Could you check a few things on this model? Use its own coordinates, in mm. Face numbers are marked on the shaded views. A direction names the side the tool comes from. Round coordinates to 2 decimals unless told otherwise and drop trailing zeros. Loops run counter-clockwise (first coordinate to the right, second up) from the corner with the lowest first, then second, coordinate; pieces in that order, holes last. Notation, with made-up numbers: (39.5, 45.5) -> (66.5, 45.5) arc R20 ccw to (66.5, 72.5) -> close; hole circle Ø10 at (1.25, 38.5). An arc over 180 degrees is marked (long way). Put each result on its own line as item: value. Start each with the question number.
1. I'm going to push flat-ended pins straight in: P1, Ø2, axis at x = 17, z = -3.5, coming from the +Y side; P2, Ø4, axis at y = -1, z = 2, coming from the +X side; P3, Ø8, axis at x = 14.5, y = -13.5, coming from the +Z side; P4, Ø4, axis at x = -0.5, y = 9, coming from the +Z side. Where does each tip first touch, or does it pass through?
2. Imagine slicing it at A-A, the plane x = 0. Please give me the cut outline in (y, z).
3. Imagine slicing it at C-C, the plane z = 3. Please give me the cut outline in (x, y), and give its area (3 significant figures).
4. Imagine slicing it at D-D, the plane x = -6. Please give me the cut outline in (y, z).
5. Which directions (+Z, -Z, +X, -X, +Y, -Y) give clear straight access to the entire face, cutting with the end or side of a thin tool? Please do the marked faces 1, 2 and 3.
6. If we mould it in two halves opening along X, with no side actions, what happens to the marked faces 4, 5 and 6? For each: pulls with the +X half, pulls with the -X half, needs draft (parallel to the pull), parting line crosses it, or undercut.
7. I need wall thicknesses on line 1 (X direction, y = -9, z = -1.5); line 2 (Y direction, x = 0, z = -3.25); line 3 (X direction, y = 7.5, z = -0.75). Which ranges of each line are inside material? Lowest first, please. Write a range as [from, to].
8. Imagine slicing it at B-B, the plane y = 0. Please give me the cut outline in (x, z).
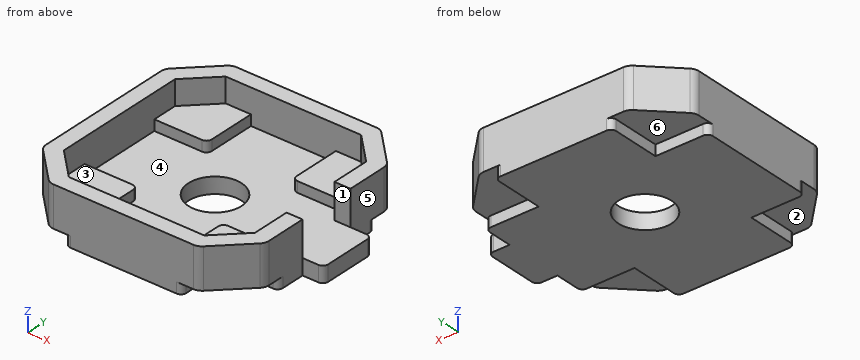
```python
from build123d import *

# Parameters (mm, degrees)
SKETCH1_W           = 42
SKETCH1_H           = 42
BOSS_EXTRUDE1_DEPTH = 4.8
CUT_EXTRUDE1_REACH  = 33.212
CUT_EXTRUDE2_DEPTH  = 2
SKETCH4_W           = 3
SKETCH4_H           = 11
BOSS_EXTRUDE2_DEPTH = 4
SHELL1_T            = -3
CUT_EXTRUDE3_REACH  = 49.202
SKETCH5_W           = 6.6
SKETCH5_H           = 11
CUT_EXTRUDE4_REACH  = 36.032
SKETCH6_R           = 5
FILLET1_R           = 2
FILLET2_R           = 1


with BuildPart() as part:
    # Sketch1 → Boss-Extrude1 (new, symmetric)
    with BuildSketch(Plane.XY):
        Rectangle(SKETCH1_W, SKETCH1_H)
    extrude(amount=BOSS_EXTRUDE1_DEPTH, both=True)

    # Sketch2 → Cut-Extrude1 (cut, up to next)
    with BuildSketch(Plane.XY.offset(4.8), mode=Mode.PRIVATE) as cut_extrude1_sk1:
        Polygon((-21, 21), (-21, 14), (-14, 21), align=None)
    cut_extrude1_tool1 = extrude(cut_extrude1_sk1.sketch, amount=-CUT_EXTRUDE1_REACH, mode=Mode.PRIVATE) & part.part
    # Sketch2 → Cut-Extrude1 (cut, up to next)
    with BuildSketch(Plane.XY.offset(4.8), mode=Mode.PRIVATE) as cut_extrude1_sk2:
        Polygon((14, 21), (21, 21), (21, 14), align=None)
    cut_extrude1_tool2 = extrude(cut_extrude1_sk2.sketch, amount=-CUT_EXTRUDE1_REACH, mode=Mode.PRIVATE) & part.part
    # Sketch2 → Cut-Extrude1 (cut, up to next)
    with BuildSketch(Plane.XY.offset(4.8), mode=Mode.PRIVATE) as cut_extrude1_sk3:
        Polygon((21, -21), (21, -14), (14, -21), align=None)
    cut_extrude1_tool3 = extrude(cut_extrude1_sk3.sketch, amount=-CUT_EXTRUDE1_REACH, mode=Mode.PRIVATE) & part.part
    # Sketch2 → Cut-Extrude1 (cut, up to next)
    with BuildSketch(Plane.XY.offset(4.8), mode=Mode.PRIVATE) as cut_extrude1_sk4:
        Polygon((-14, -21), (-21, -21), (-21, -14), align=None)
    cut_extrude1_tool4 = extrude(cut_extrude1_sk4.sketch, amount=-CUT_EXTRUDE1_REACH, mode=Mode.PRIVATE) & part.part
    add(cut_extrude1_tool1.solids().sort_by_distance((-18.666667, 18.666667, 4.8))[0], mode=Mode.SUBTRACT)
    add(cut_extrude1_tool2.solids().sort_by_distance((18.666667, 18.666667, 4.8))[0], mode=Mode.SUBTRACT)
    add(cut_extrude1_tool3.solids().sort_by_distance((18.666667, -18.666667, 4.8))[0], mode=Mode.SUBTRACT)
    add(cut_extrude1_tool4.solids().sort_by_distance((-18.666667, -18.666667, 4.8))[0], mode=Mode.SUBTRACT)

    # Sketch3 → Cut-Extrude2 (cut)
    with BuildSketch(Plane(origin=(0, 0, -4.8), x_dir=(-1, 0, 0), z_dir=(0, 0, -1))):
        Polygon((-21, 14), (-21, 11), (-11, 11), (-11, 21), (-14, 21), align=None)
        Polygon((14, 21), (11, 21), (11, 11), (21, 11), (21, 14), align=None)
        Polygon((11, -11), (11, -21), (14, -21), (21, -14), (21, -11), align=None)
        Polygon((-11, -11), (-21, -11), (-21, -14), (-14, -21), (-11, -21), align=None)
    extrude(amount=-CUT_EXTRUDE2_DEPTH, mode=Mode.SUBTRACT)

    # Sketch4 → Boss-Extrude2 (add)
    with BuildSketch(Plane(origin=(21, 0, 0), x_dir=(0, 0, -1), z_dir=(1, 0, 0))):
        with Locations((3.3, 0)):
            Rectangle(SKETCH4_W, SKETCH4_H)
    extrude(amount=BOSS_EXTRUDE2_DEPTH)

    # Shell1
    shell1_openings = [part.faces().sort_by_distance(p)[0] for p in [
        (0, 0, 4.8),
    ]]
    offset(amount=SHELL1_T, openings=shell1_openings, kind=Kind.INTERSECTION)

    # Sketch5 → Cut-Extrude3 (cut, up to next)
    with BuildSketch(Plane(origin=(21, 0, 0), x_dir=(0, 0, -1), z_dir=(1, 0, 0)), mode=Mode.PRIVATE) as cut_extrude3_sk1:
        with Locations((-1.5, 0)):
            Rectangle(SKETCH5_W, SKETCH5_H)
    cut_extrude3_tool1 = extrude(cut_extrude3_sk1.sketch, amount=-CUT_EXTRUDE3_REACH, mode=Mode.PRIVATE) & part.part
    add(cut_extrude3_tool1.solids().sort_by_distance((21, 0, 1.5))[0], mode=Mode.SUBTRACT)

    # Sketch6 → Cut-Extrude4 (cut, up to next)
    with BuildSketch(Plane(origin=(0, 0, -4.8), x_dir=(-1, 0, 0), z_dir=(0, 0, -1)), mode=Mode.PRIVATE) as cut_extrude4_sk1:
        Circle(SKETCH6_R)
    cut_extrude4_tool1 = extrude(cut_extrude4_sk1.sketch, amount=-CUT_EXTRUDE4_REACH, mode=Mode.PRIVATE) & part.part
    add(cut_extrude4_tool1.solids().sort_by_distance((0, 0, -4.8))[0], mode=Mode.SUBTRACT)

    # Fillet1
    fillet1_edges = [part.edges().sort_by_distance(p)[0] for p in [
        (-14, -21, 1),
        (-21, -14, 1),
        (21, -14, 1),
        (14, -21, 1),
        (14, 21, 1),
        (21, 14, 1),
        (-21, 14, 1),
        (-14, 21, 1),
    ]]
    fillet(fillet1_edges, radius=FILLET1_R)

    # Fillet2
    fillet2_edges = [part.edges().sort_by_distance(p)[0] for p in [
        (25, 5.5, -3.3),
        (25, -5.5, -3.3),
        (-8, -8, -0.8),
        (8, -8, -0.8),
        (8, 8, -0.8),
        (-8, 8, -0.8),
        (21, -11, -3.8),
        (11, -21, -3.8),
        (-11, -21, -3.8),
        (-21, -11, -3.8),
        (-21, 11, -3.8),
        (-11, 21, -3.8),
        (11, 21, -3.8),
        (21, 11, -3.8),
    ]]
    fillet(fillet2_edges, radius=FILLET2_R)


solid = part.part
```
Entries:
1. P1: y = 18.71
1. P2: x = -18
1. P3: z = 4.8
1. P4: z = -1.8
2. outline: (-21, -4.8) -> (-5, -4.8) -> (-5, -1.8) -> (-18, -1.8) -> (-18, 4.8) -> (-21, 4.8) -> close; (5, -4.8) -> (21, -4.8) -> (21, 4.8) -> (18, 4.8) -> (18, -1.8) -> (5, -1.8) -> close
3. outline: (-21, -13.17) arc R2 ccw to (-20.41, -14.59) -> (-14.59, -20.41) arc R2 ccw to (-13.17, -21) -> (13.17, -21) arc R2 ccw to (14.59, -20.41) -> (20.41, -14.59) arc R2 ccw to (21, -13.17) -> (21, -5.5) -> (18, -5.5) -> (18, -12.76) -> (12.76, -18) -> (-12.76, -18) -> (-18, -12.76) -> (-18, 12.76) -> (-12.76, 18) -> (12.76, 18) -> (18, 12.76) -> (18, 5.5) -> (21, 5.5) -> (21, 13.17) arc R2 ccw to (20.41, 14.59) -> (14.59, 20.41) arc R2 ccw to (13.17, 21) -> (-13.17, 21) arc R2 ccw to (-14.59, 20.41) -> (-20.41, 14.59) arc R2 ccw to (-21, 13.17) -> close
3. area: 391 mm^2
4. outline: (-21, -4.8) -> (21, -4.8) -> (21, 4.8) -> (18, 4.8) -> (18, -1.8) -> (-18, -1.8) -> (-18, 4.8) -> (-21, 4.8) -> close
5. face 1: +Z, +X
5. face 2: -Z, -X, -Y
5. face 3: +Z
6. face 4: undercut
6. face 5: pulls with the +X half
6. face 6: needs draft
7. line 1: [-21, -8], [8, 21]
7. line 2: [-21, -5], [5, 21]
7. line 3: [-21, -18], [18, 21]
8. outline: (-21, -4.8) -> (-5, -4.8) -> (-5, -1.8) -> (-18, -1.8) -> (-18, 4.8) -> (-21, 4.8) -> close; (5, -4.8) -> (25, -4.8) -> (25, -1.8) -> (5, -1.8) -> close
